The figure shows three views and two pictorial views of one solid part (mm, origin at its lowest corner). Answer the questions. A direction names the side the tool comes from. Give positions to 0.01 mm unless a question says otherwise; leave off trailing zeros. Write each loop counter-clockwise with the first axis right and the second up, starting at its lowest first coordinate (ties: lowest second). Pieces come first, ordered by that corner, then holes. Notation, with made-up numbers: (73.5, -17.5) -> (88.5, -17.5) arc R25 ccw to (88.5, 11.5) -> close; hole circle Ø2 at (39, 64). An arc over 180 degrees is marked (long way). Answer as CSV lines item,"result". Start each with the question number.
1. The part is cut by section B-B, the plane z = 21.5. Determine the outline of the cut face in (x, y), and give its area (3 significant figures).
2. The part is cut by section D-D, the plane y = 23. Determine the outline of the cut face in (x, z).
3. Given pin 1 (6 mm diameter, centred on x = 20.5, z = 16, fed in from -Y); pin 2 (1.5 mm diameter, centred on x = 20.5, z = 18.5, fed in from -Y); pin 3 (6 mm diameter, centred on x = 17, z = 8, fed in from -Y), each flat-ended and moving along its own axis, determine where each tip first touches the part or whether it passes through.
4. For a pull along X with two mould halves and no side action, classify the marked faces 1, 2 and 3 as pulls with the +X half, pulls with the -X half, needs draft (parallel to the pull), parting line crosses it, or undercut.
5. Find the intervals of material crossed by line 1 (X direction, y = 13.5, z = 12) (1 decimal); line 2 (X direction, y = 7.5, z = 3.75) (1 decimal); line 3 (Y direction, x = 16, z = 12.5), in increasing order.
6. The part is cut by section A-A, the plane x = 12.7. Determine the outline of the cut face in (y, z).
7. The part is cut by section C-C, the plane y = 13.75. Determine the outline of the cut face in (x, z).
8. A tool of negligible diameter and unlimited length cuts with its end or side. For the marked faces 4 and 5, from which of +Z, -Z, +X, -X, +Y, -Y can it reach the whole face along a straight path? Write none if from no direction.
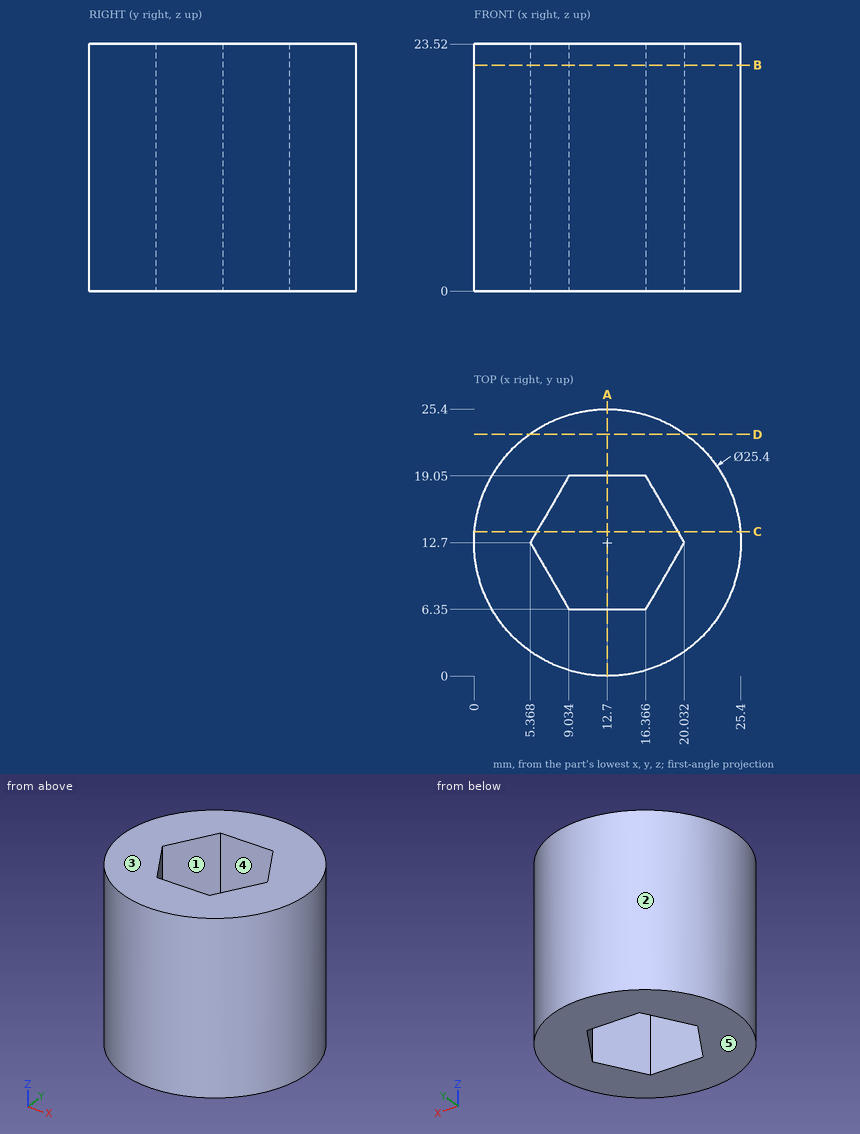
Results found:
1,outline,"circle Ø25.4 at (12.7, 12.7); hole (5.37, 12.7) -> (9.03, 6.35) -> (16.37, 6.35) -> (20.03, 12.7) -> (16.37, 19.05) -> (9.03, 19.05) -> close"
1,area,"367 mm²"
2,outline,"(5.27, 0) -> (20.13, 0) -> (20.13, 23.52) -> (5.27, 23.52) -> close"
3,pin 1,"stops at y = 0.94"
3,pin 2,"stops at y = 2.14"
3,pin 3,"stops at y = 0.07"
4,face 1,"undercut"
4,face 2,"parting line crosses it"
4,face 3,"needs draft"
5,line 1,"x = 0 to 5.8, 19.6 to 25.4"
5,line 2,"x = 1.1 to 8.4, 17 to 24.3"
5,line 3,"y = 0.44 to 6.35, 19.05 to 24.96"
6,outline,"(0, 0) -> (6.35, 0) -> (6.35, 23.52) -> (0, 23.52) -> close; (19.05, 0) -> (25.4, 0) -> (25.4, 23.52) -> (19.05, 23.52) -> close"
7,outline,"(0.04, 0) -> (5.97, 0) -> (5.97, 23.52) -> (0.04, 23.52) -> close; (19.43, 0) -> (25.36, 0) -> (25.36, 23.52) -> (19.43, 23.52) -> close"
8,face 4,"+Z, -Z"
8,face 5,"-Z, +X, -X, +Y, -Y"
